For this review, take the finished solid that the model builds, in its own axes (mm). Round coordinates to 2 decimals unless told otherwise and drop trailing zeros. Write each loop counter-clockwise with the first axis right and the second up, starting at its lowest first coordinate (ties: lowest second). Pieces come first, ordered by that corner, then holes. Notation, with made-up numbers: (9.25, 43) - (46.25, 43) arc R12 cw to (46.25, 62) - close; hole circle Ø2 at (-24, 13). An arc over 180 degrees is marked (long way). Answer in a Markdown table with one row per item. Add a question column.
from build123d import *

# Parameters (mm, degrees)
SKETCH1_W                     = 110
SKETCH1_H                     = 160
BOSS_EXTRUDE1_DEPTH           = 10
BOSS_EXTRUDE1_DRAFT           = -2
SHELL1_T                      = -2
SKETCH3_W                     = 108.69841539
SKETCH3_H                     = 158.69841539
CUT_EXTRUDE3_DEPTH            = 5
CUT_EXTRUDE3_DRAFT            = -2
SKETCH4_W                     = 71
SKETCH4_H                     = 23.8
CUT_EXTRUDE4_DEPTH            = 2
CUT_EXTRUDE4_DRAFT            = 2
SKETCH10_R                    = 0.75
BOSS_EXTRUDE3_DEPTH           = 3
BOSS_EXTRUDE3_DRAFT           = 2
BOSS_EXTRUDE3_PROFILE_2_DEPTH = 3
BOSS_EXTRUDE3_PROFILE_2_DRAFT = 2
BOSS_EXTRUDE3_PROFILE_3_DEPTH = 3
BOSS_EXTRUDE3_PROFILE_3_DRAFT = 2
BOSS_EXTRUDE3_PROFILE_4_DEPTH = 3
BOSS_EXTRUDE3_PROFILE_4_DRAFT = 2
SKETCH13_W                    = 5
SKETCH13_H                    = 10
BOSS_EXTRUDE8_DEPTH           = 20
BOSS_EXTRUDE8_DRAFT           = 2
BOSS_EXTRUDE8_PROFILE_2_DEPTH = 20
BOSS_EXTRUDE8_PROFILE_2_DRAFT = 2
CUT_EXTRUDE8_REACH            = 138.446
SKETCH21_R                    = 2
CUT_EXTRUDE8_DRAFT            = -2
CUT_EXTRUDE9_REACH            = 138.446
SKETCH22_R                    = 2
CUT_EXTRUDE9_DRAFT            = -2
SKETCH27_W                    = 69
SKETCH27_H                    = 76
CUT_EXTRUDE10_DEPTH           = 1
CUT_EXTRUDE10_DRAFT           = -2
SKETCH28_W                    = 25
SKETCH28_H                    = 5
CUT_EXTRUDE11_DEPTH           = 1
CUT_EXTRUDE11_DRAFT           = -2


with BuildPart() as part:
    # Sketch1 → Boss-Extrude1 (with draft: the straight prism first)
    with BuildSketch(Plane.XY):
        Rectangle(SKETCH1_W, SKETCH1_H)
    extrude(amount=BOSS_EXTRUDE1_DEPTH)
    # Boss-Extrude1: the draft: its side faces are tilted about the plane it starts from
    boss_extrude1_sides = [part.faces().sort_by_distance(p)[0] for p in [
        (55, 0, 5),
        (0, 80, 5),
        (-55, 0, 5),
        (0, -80, 5),
    ]]
    draft(boss_extrude1_sides, Plane.XY, BOSS_EXTRUDE1_DRAFT)

    # Shell1
    shell1_openings = [part.faces().sort_by_distance(p)[0] for p in [
        (0, 0, 10),
    ]]
    offset(amount=SHELL1_T, openings=shell1_openings, kind=Kind.INTERSECTION)


with BuildPart() as cut_extrude3_tool:
    # Sketch3 → Cut-Extrude3 (with draft: the straight prism first)
    with BuildSketch(Plane.XY.offset(10)):
        Rectangle(SKETCH3_W, SKETCH3_H)
    extrude(amount=-CUT_EXTRUDE3_DEPTH)
    # Cut-Extrude3: the draft: its side faces are tilted about the plane it starts from
    cut_extrude3_sides = [cut_extrude3_tool.faces().sort_by_distance(p)[0] for p in [
        (54.349207695, 0, 7.5),
        (0, 79.349207695, 7.5),
        (-54.349207695, 0, 7.5),
        (0, -79.349207695, 7.5),
    ]]
    draft(cut_extrude3_sides, Plane.XY.offset(10), CUT_EXTRUDE3_DRAFT)


with BuildPart() as part_1:
    add(part.part)

    # Cut-Extrude3: cut by cut_extrude3_tool
    add(cut_extrude3_tool.part, mode=Mode.SUBTRACT)


with BuildPart() as cut_extrude4_tool:
    # Sketch4 → Cut-Extrude4 (with draft: the straight prism first)
    with BuildSketch(Plane(origin=(0, 0, 0), x_dir=(-1, 0, 0), z_dir=(0, 0, -1))):
        with Locations((0, 43.1)):
            Rectangle(SKETCH4_W, SKETCH4_H)
    extrude(amount=-CUT_EXTRUDE4_DEPTH)
    # Cut-Extrude4: the draft: its side faces are tilted about the plane it starts from
    cut_extrude4_sides = [cut_extrude4_tool.faces().sort_by_distance(p)[0] for p in [
        (-35.5, 43.1, 1),
        (0, 55, 1),
        (35.5, 43.1, 1),
        (0, 31.2, 1),
    ]]
    draft(cut_extrude4_sides, Plane(origin=(0, 0, 0), x_dir=(-1, 0, 0), z_dir=(0, 0, -1)), CUT_EXTRUDE4_DRAFT)


with BuildPart() as part_2:
    add(part_1.part)

    # Cut-Extrude4: cut by cut_extrude4_tool
    add(cut_extrude4_tool.part, mode=Mode.SUBTRACT)


with BuildPart() as boss_extrude3_tool:
    # Sketch10 → Boss-Extrude3 (with draft: the straight prism first)
    with BuildSketch(Plane.XY.offset(2)):
        with Locations((-37.569841539, 57.294841539)):
            Circle(SKETCH10_R)
    extrude(amount=BOSS_EXTRUDE3_DEPTH)
    # Boss-Extrude3: the draft: its side faces are tilted about the plane it starts from
    boss_extrude3_sides = [boss_extrude3_tool.faces().sort_by_distance(p)[0] for p in [
        (-38.319841539, 57.294841539, 3.5),
    ]]
    draft(boss_extrude3_sides, Plane.XY.offset(2), BOSS_EXTRUDE3_DRAFT)


with BuildPart() as part_3:
    add(part_2.part)

    # Boss-Extrude3: add boss_extrude3_tool
    add(boss_extrude3_tool.part)


with BuildPart() as boss_extrude3_profile_2_tool:
    # Sketch10 → Boss-Extrude3 profile 2 (with draft: the straight prism first)
    with BuildSketch(Plane.XY.offset(2)):
        with Locations((37.430158461, 57.294841539)):
            Circle(SKETCH10_R)
    extrude(amount=BOSS_EXTRUDE3_PROFILE_2_DEPTH)
    # Boss-Extrude3 profile 2: the draft: its side faces are tilted about the plane it starts from
    boss_extrude3_profile_2_sides = [boss_extrude3_profile_2_tool.faces().sort_by_distance(p)[0] for p in [
        (36.680158461, 57.294841539, 3.5),
    ]]
    draft(boss_extrude3_profile_2_sides, Plane.XY.offset(2), BOSS_EXTRUDE3_PROFILE_2_DRAFT)


with BuildPart() as part_4:
    add(part_3.part)

    # Boss-Extrude3 profile 2: add boss_extrude3_profile_2_tool
    add(boss_extrude3_profile_2_tool.part)


with BuildPart() as boss_extrude3_profile_3_tool:
    # Sketch10 → Boss-Extrude3 profile 3 (with draft: the straight prism first)
    with BuildSketch(Plane.XY.offset(2)):
        with Locations((37.430158461, 26.294841539)):
            Circle(SKETCH10_R)
    extrude(amount=BOSS_EXTRUDE3_PROFILE_3_DEPTH)
    # Boss-Extrude3 profile 3: the draft: its side faces are tilted about the plane it starts from
    boss_extrude3_profile_3_sides = [boss_extrude3_profile_3_tool.faces().sort_by_distance(p)[0] for p in [
        (36.680158461, 26.294841539, 3.5),
    ]]
    draft(boss_extrude3_profile_3_sides, Plane.XY.offset(2), BOSS_EXTRUDE3_PROFILE_3_DRAFT)


with BuildPart() as part_5:
    add(part_4.part)

    # Boss-Extrude3 profile 3: add boss_extrude3_profile_3_tool
    add(boss_extrude3_profile_3_tool.part)


with BuildPart() as boss_extrude3_profile_4_tool:
    # Sketch10 → Boss-Extrude3 profile 4 (with draft: the straight prism first)
    with BuildSketch(Plane.XY.offset(2)):
        with Locations((-37.569841539, 26.294841539)):
            Circle(SKETCH10_R)
    extrude(amount=BOSS_EXTRUDE3_PROFILE_4_DEPTH)
    # Boss-Extrude3 profile 4: the draft: its side faces are tilted about the plane it starts from
    boss_extrude3_profile_4_sides = [boss_extrude3_profile_4_tool.faces().sort_by_distance(p)[0] for p in [
        (-38.319841539, 26.294841539, 3.5),
    ]]
    draft(boss_extrude3_profile_4_sides, Plane.XY.offset(2), BOSS_EXTRUDE3_PROFILE_4_DRAFT)


with BuildPart() as part_6:
    add(part_5.part)

    # Boss-Extrude3 profile 4: add boss_extrude3_profile_4_tool
    add(boss_extrude3_profile_4_tool.part)


with BuildPart() as boss_extrude8_tool:
    # Sketch13 → Boss-Extrude8 (with draft: the straight prism first)
    with BuildSketch(Plane.XY.offset(2)):
        with Locations((-50.56862245, 0)):
            Rectangle(SKETCH13_W, SKETCH13_H)
    extrude(amount=BOSS_EXTRUDE8_DEPTH)
    # Boss-Extrude8: the draft: its side faces are tilted about the plane it starts from
    boss_extrude8_sides = [boss_extrude8_tool.faces().sort_by_distance(p)[0] for p in [
        (-50.56862245, 5, 12),
        (-53.06862245, 0, 12),
        (-50.56862245, -5, 12),
        (-48.06862245, 0, 12),
    ]]
    draft(boss_extrude8_sides, Plane.XY.offset(2), BOSS_EXTRUDE8_DRAFT)


with BuildPart() as part_7:
    add(part_6.part)

    # Boss-Extrude8: add boss_extrude8_tool
    add(boss_extrude8_tool.part)


with BuildPart() as boss_extrude8_profile_2_tool:
    # Sketch13 → Boss-Extrude8 profile 2 (with draft: the straight prism first)
    with BuildSketch(Plane.XY.offset(2)):
        with Locations((50.56862245, 0)):
            Rectangle(SKETCH13_W, SKETCH13_H)
    extrude(amount=BOSS_EXTRUDE8_PROFILE_2_DEPTH)
    # Boss-Extrude8 profile 2: the draft: its side faces are tilted about the plane it starts from
    boss_extrude8_profile_2_sides = [boss_extrude8_profile_2_tool.faces().sort_by_distance(p)[0] for p in [
        (50.56862245, -5, 12),
        (53.06862245, 0, 12),
        (50.56862245, 5, 12),
        (48.06862245, 0, 12),
    ]]
    draft(boss_extrude8_profile_2_sides, Plane.XY.offset(2), BOSS_EXTRUDE8_PROFILE_2_DRAFT)


with BuildPart() as part_8:
    add(part_7.part)

    # Boss-Extrude8 profile 2: add boss_extrude8_profile_2_tool
    add(boss_extrude8_profile_2_tool.part)

    # Cut-Extrude8: up to this plane
    cut_extrude8_end = Plane(origin=(-48.06862245, 5, 2), z_dir=(0.9993908270190958, 0, 0.034899496702501004))



with BuildPart() as cut_extrude8_long_prism_1:
    # Sketch21 → Cut-Extrude8 (the long prism of profile 1, to be tilted and cut off)
    with BuildSketch(Plane(origin=(-53.073742676, 0, 1.853375934), x_dir=(0.03489949670250101, 0, 0.9993908270190958), z_dir=(-0.9993908270190958, 0, 0.03489949670250101))):
        with Locations((15.062248779, 0)):
            Circle(SKETCH21_R)
    extrude(amount=-CUT_EXTRUDE8_REACH)
    cut_extrude8_tool1_sides = [cut_extrude8_long_prism_1.faces().sort_by_distance(p)[0] for p in [
        (16.562954451, 0, 12.491819684),
    ]]
    draft(cut_extrude8_tool1_sides, Plane(origin=(-53.073742676, 0, 1.853375934), x_dir=(0.03489949670250101, 0, 0.9993908270190958), z_dir=(-0.9993908270190958, 0, 0.03489949670250101)), CUT_EXTRUDE8_DRAFT)  # the draft: side faces tilted about the start plane


with BuildPart() as part_9:
    add(part_8.part)
    cut_extrude8_tool1 = split(cut_extrude8_long_prism_1.part, bisect_by=cut_extrude8_end, keep=Keep.BOTH, mode=Mode.PRIVATE)
    add(cut_extrude8_tool1.solids().sort_by_distance((-52.548078, 0, 16.906449))[0], mode=Mode.SUBTRACT)

    # Cut-Extrude9: up to this plane
    cut_extrude9_end = Plane(origin=(48.06862245, -5, 2), z_dir=(-0.9993908270190958, 0, 0.034899496702501004))



with BuildPart() as cut_extrude9_long_prism_1:
    # Sketch22 → Cut-Extrude9 (the long prism of profile 1, to be tilted and cut off)
    with BuildSketch(Plane(origin=(53.073742676, 0, 1.853375934), x_dir=(0.03489949670250101, 0, -0.9993908270190958), z_dir=(0.9993908270190958, 0, 0.03489949670250101))):
        with Locations((-15.062248779, 0)):
            Circle(SKETCH22_R)
    extrude(amount=-CUT_EXTRUDE9_REACH)
    cut_extrude9_tool1_sides = [cut_extrude9_long_prism_1.faces().sort_by_distance(p)[0] for p in [
        (-16.702552438, 0, 16.489382992),
    ]]
    draft(cut_extrude9_tool1_sides, Plane(origin=(53.073742676, 0, 1.853375934), x_dir=(0.03489949670250101, 0, -0.9993908270190958), z_dir=(0.9993908270190958, 0, 0.03489949670250101)), CUT_EXTRUDE9_DRAFT)  # the draft: side faces tilted about the start plane


with BuildPart() as part_10:
    add(part_9.part)
    cut_extrude9_tool1 = split(cut_extrude9_long_prism_1.part, bisect_by=cut_extrude9_end, keep=Keep.BOTH, mode=Mode.PRIVATE)
    add(cut_extrude9_tool1.solids().sort_by_distance((52.548078, 0, 16.906449))[0], mode=Mode.SUBTRACT)


with BuildPart() as cut_extrude10_tool:
    # Sketch27 → Cut-Extrude10 (with draft: the straight prism first)
    with BuildSketch(Plane(origin=(0, 0, 0), x_dir=(-1, 0, 0), z_dir=(0, 0, -1))):
        with Locations((5.5, -31.8)):
            Rectangle(SKETCH27_W, SKETCH27_H)
    extrude(amount=-CUT_EXTRUDE10_DEPTH)
    # Cut-Extrude10: the draft: its side faces are tilted about the plane it starts from
    cut_extrude10_sides = [cut_extrude10_tool.faces().sort_by_distance(p)[0] for p in [
        (-40, -31.8, 0.5),
        (-5.5, 6.2, 0.5),
        (29, -31.8, 0.5),
        (-5.5, -69.8, 0.5),
    ]]
    draft(cut_extrude10_sides, Plane(origin=(0, 0, 0), x_dir=(-1, 0, 0), z_dir=(0, 0, -1)), CUT_EXTRUDE10_DRAFT)


with BuildPart() as part_11:
    add(part_10.part)

    # Cut-Extrude10: cut by cut_extrude10_tool
    add(cut_extrude10_tool.part, mode=Mode.SUBTRACT)


with BuildPart() as cut_extrude11_tool:
    # Sketch28 → Cut-Extrude11 (with draft: the straight prism first)
    with BuildSketch(Plane(origin=(0, 0, 1), x_dir=(-1, 0, 0), z_dir=(0, 0, -1))):
        with Locations((6.534920769, -62.465079231)):
            Rectangle(SKETCH28_W, SKETCH28_H)
    extrude(amount=-CUT_EXTRUDE11_DEPTH)
    # Cut-Extrude11: the draft: its side faces are tilted about the plane it starts from
    cut_extrude11_sides = [cut_extrude11_tool.faces().sort_by_distance(p)[0] for p in [
        (-6.534920769, -59.965079231, 1.5),
        (5.965079231, -62.465079231, 1.5),
        (-6.534920769, -64.965079231, 1.5),
        (-19.034920769, -62.465079231, 1.5),
    ]]
    draft(cut_extrude11_sides, Plane(origin=(0, 0, 1), x_dir=(-1, 0, 0), z_dir=(0, 0, -1)), CUT_EXTRUDE11_DRAFT)


with BuildPart() as part_12:
    add(part_11.part)

    # Cut-Extrude11: cut by cut_extrude11_tool
    add(cut_extrude11_tool.part, mode=Mode.SUBTRACT)


solid = part_12.part
Q1. To check wall thickness, follow probe 1 along Y at (x, z) = (10, 9.25); probe 2 along X at (y, z) = (-32.5, 7.5); probe 3 along Z at (x, y) = (-19, -58.5). State the ranges of each line that lie inside material, in increasing order.
Q2. Add section D-D on z = 8. State the section outline as (x, y) points.
Q3. Add section A-A on y = 37.5. State the section outline as (x, z) points, then the cut area to 3 significant figures.
Q4. Draft analysis for pull direction Y (two halves, no side actions). For faces 1 (the face through (-51, 0, 22)), 2 (the face through (50.592, -0.739, 15.055)), 3 (the face through (-1, 1, 2)), state which applies: released by +Y, released by -Y, zero draft, split by the parting line, or undercut.
Q5. Add section C-C on x = -7. State the section outline as (y, z) points.
Q6. Insertion check: pin 1 Ø10 at (y, z) = (25.5, 6.5) entering from -X; pin 2 Ø0.6 at (x, y) = (37.5, 57) entering from +Z; pin 3 Ø1.5 at (x, z) = (-28, 5.5) entering from -Y; pin 4 Ø4 at (y, z) = (1, 6.5) entering from +X. Each pin has a flat end and moves straight along its axis. Give the tip position at first contact, or say it passes through.
Q7. Add section B-B on x = 22. State the section outline as (y, z) points, then the cut area to 3 significant figures.
Answer sheet:
| question | item | result |
|---|---|---|
| 1 | probe 1 | y = -80.32 to -79.32, 79.32 to 80.32 |
| 1 | probe 2 | x = -55.26 to -54.26, 54.26 to 55.26 |
| 1 | probe 3 | z = 1 to 2 |
| 2 | outline | (-55.28, -80.28) - (55.28, -80.28) - (55.28, 80.28) - (-55.28, 80.28) - close; (-52.86, -4.79) - (-48.28, -4.79) - (-48.28, 4.79) - (-52.86, 4.79) - close; (48.28, -4.79) - (52.86, -4.79) - (52.86, 4.79) - (48.28, 4.79) - close; hole (-54.28, -79.28) - (54.28, -79.28) - (54.28, 79.28) - (-54.28, 79.28) - close |
| 3 | outline | (-55.35, 10) - (-55, 0) - (-35.5, 0) - (-35.57, 2) - (-53.07, 2) - (-53.17, 5) - (-54.17, 5) - (-54.35, 10) - close; (35.5, 0) - (55, 0) - (55.35, 10) - (54.35, 10) - (54.17, 5) - (53.17, 5) - (53.07, 2) - (35.57, 2) - close |
| 3 | area | 100 mm² |
| 4 | face 1 | zero draft |
| 4 | face 2 | undercut |
| 4 | face 3 | undercut |
| 5 | outline | (-80.35, 10) - (-80, 0) - (-69.8, 0) - (-69.77, 1) - (-64.97, 1) - (-64.93, 2) - (-78.07, 2) - (-78.17, 5) - (-79.17, 5) - (-79.35, 10) - close; (-60, 2) - (-59.97, 1) - (6.17, 1) - (6.2, 0) - (31.2, 0) - (31.13, 2) - close; (55, 0) - (80, 0) - (80.35, 10) - (79.35, 10) - (79.17, 5) - (78.17, 5) - (78.07, 2) - (55.07, 2) - close |
| 6 | pin 1 | stops at x = -55.35 |
| 6 | pin 2 | stops at z = 5 |
| 6 | pin 3 | stops at y = -80.22 |
| 6 | pin 4 | stops at x = 55.3 |
| 7 | outline | (-80.35, 10) - (-80, 0) - (-69.8, 0) - (-69.77, 1) - (6.17, 1) - (6.2, 0) - (31.2, 0) - (31.13, 2) - (-78.07, 2) - (-78.17, 5) - (-79.17, 5) - (-79.35, 10) - close; (55, 0) - (80, 0) - (80.35, 10) - (79.35, 10) - (79.17, 5) - (78.17, 5) - (78.07, 2) - (55.07, 2) - close |
| 7 | area | 218 mm² |
